```python
from build123d import *

# Parameters (mm, degrees)
F0_W     = 113.5
F0_H     = 50.5
F1_DEPTH = 215
F3_DEPTH = 113.501
F4_W     = 109.5
F4_H     = 18
F5_DEPTH = 43
F6_R     = 1.595
F7_DEPTH = 113.501
F8_R     = 1.595
F9_DEPTH = 10


with BuildPart() as f1:
    # F0 (on Top) → F1 (new body)
    with BuildSketch(Plane.XY):
        with Locations((56.75, 25.25)):
            Rectangle(F0_W, F0_H)
    extrude(amount=F1_DEPTH)

    # F2 (on face) → F3 (cut, through all)
    with BuildSketch(Plane.YZ.offset(113.5)):
        with BuildLine():
            Line((36.05, 209.85), (14.45, 209.85))
            ThreePointArc((14.45, 209.85), (13.38934, 209.41066), (12.95, 208.35))
            ThreePointArc((12.95, 208.35), (13.38934, 207.28934), (14.45, 206.85))
            Line((14.45, 206.85), (36.05, 206.85))
            ThreePointArc((36.05, 206.85), (37.11066, 207.28934), (37.55, 208.35))
            ThreePointArc((37.55, 208.35), (37.11066, 209.41066), (36.05, 209.85))
        make_face()
        with BuildLine():
            ThreePointArc((12.95, 201.35), (13.38934, 200.28934), (14.45, 199.85))
            Line((14.45, 199.85), (36.05, 199.85))
            ThreePointArc((36.05, 199.85), (37.11066, 200.28934), (37.55, 201.35))
            ThreePointArc((37.55, 201.35), (37.11066, 202.41066), (36.05, 202.85))
            Line((36.05, 202.85), (14.45, 202.85))
            ThreePointArc((14.45, 202.85), (13.38934, 202.41066), (12.95, 201.35))
        make_face()
        with BuildLine():
            ThreePointArc((12.95, 194.35), (13.38934, 193.28934), (14.45, 192.85))
            Line((14.45, 192.85), (36.05, 192.85))
            ThreePointArc((36.05, 192.85), (37.11066, 193.28934), (37.55, 194.35))
            ThreePointArc((37.55, 194.35), (37.11066, 195.41066), (36.05, 195.85))
            Line((36.05, 195.85), (14.45, 195.85))
            ThreePointArc((14.45, 195.85), (13.38934, 195.41066), (12.95, 194.35))
        make_face()
    extrude(amount=-F3_DEPTH, mode=Mode.SUBTRACT)

    # F4 (on face) → F5 (cut)
    with BuildSketch(Plane.XZ):
        with Locations((56.75, 206)):
            Rectangle(F4_W, F4_H)
    extrude(amount=-F5_DEPTH, mode=Mode.SUBTRACT)

    # F6 (on face) → F7 (cut, through all)
    with BuildSketch(Plane.YZ.offset(113.5)):
        with Locations((39.155, 31.595)):
            Circle(F6_R)
        with Locations((39.155, 182.905)):
            Circle(F6_R)
    extrude(amount=-F7_DEPTH, mode=Mode.SUBTRACT)

    # F8 (on face) → F9 (cut)
    with BuildSketch(Plane(origin=(0, 0, 0), x_dir=(0, -1, 0), z_dir=(-1, 0, 0))):
        with Locations((-13.345, 182.905)):
            Circle(F8_R)
        with Locations((-13.345, 31.595)):
            Circle(F8_R)
    extrude(amount=-F9_DEPTH, mode=Mode.SUBTRACT)


solid = f1.part
```
Can you work these out from the model? Positions are in its coordinate system, mm. A direction names the side the tool comes from. Give positions to 0.01 mm unless a question says otherwise; leave off trailing zeros. Order: outer loops, then holes, each group sorted by start corner. A loop starts at its lowest first (then second) coordinate and runs counter-clockwise, first axis right, second up. Notation, with made-up numbers: (-33, -29) - (-21, -29) arc R19 cw to (-21, -21) - close; hole circle Ø1 at (42.5, -22). An arc over 180 degrees is marked (long way). Use a Markdown table: item, result. Add a question column.
Q1. If we mould it in two halves opening along X, with no side actions, what happens to faces 1 (the flat face through (56, 21, 197)), 2 (the flat face through (58, 25, 195.85)), 3 (the flat face through (113.5, 25, 106))? For each: released by +X, released by -X, zero draft, split by the parting line, or undercut.
Q2. I'm going to push flat-ended pins straight in: pin 1 (1.6 mm diameter, centred on y = 13, z = 183, fed in from -X); pin 2 (6.5 mm diameter, centred on x = 44, y = 21.5, fed in from +Z). Where does each tip first touch, or does it pass through?
Q3. On a 3-axis mill with a long thin cutter (end or side, diameter ignored), from which of +Z, -Z, +X, -X, +Y, -Y can I reach the whole of each face in a straight line? I mean faces 4 (the flat face through (2, 21, 206)), 5 (the flat face through (0, 25, 106)), 6 (the flat face through (58, 25, 192.85)). Say none if no direction works.
Q4. If we section it at C-C on y = 4.5: Write out the boundary of the cut face in (x, z), plus the area to 3 significant figures.
Q5. Please list where these lines run through material, in increasing order: line 1 along X through (y, z) = (37.5, 202.5); line 2 along Z through (x, y) = (82.5, 35.5); line 3 along Z through (x, y) = (86, 38) (3 decimals).
Q6. If we section it at B-B on x = 53.5: Write out the boundary of the cut face in (y, z) (3 decimals), plus the area to 4 significant figures.
Q7. If we section it at A-A on y = 19.5: Write out the boundary of the cut face in (x, z).
Answers follow:
| question | item | result |
|---|---|---|
| 1 | face 1 | undercut |
| 1 | face 2 | zero draft |
| 1 | face 3 | released by +X |
| 2 | pin 1 | stops at x = 10 |
| 2 | pin 2 | stops at z = 197 |
| 3 | face 4 | +Z, -Y |
| 3 | face 5 | +Z, -Z, -X, +Y, -Y |
| 3 | face 6 | +X, -X |
| 4 | outline | (0, 0) - (113.5, 0) - (113.5, 215) - (111.5, 215) - (111.5, 197) - (2, 197) - (2, 215) - (0, 215) - close |
| 4 | area | 22,400 mm^2 |
| 5 | line 1 | x = 0 to 2, 111.5 to 113.5 |
| 5 | line 2 | z = 0 to 192.85, 195.85 to 197 |
| 5 | line 3 | z = 0 to 30.495, 32.695 to 181.805, 184.005 to 197 |
| 6 | outline | (0, 0) - (50.5, 0) - (50.5, 215) - (43, 215) - (43, 197) - (0, 197) - close; hole (12.95, 194.35) arc R1.5 ccw to (14.45, 192.85) - (36.05, 192.85) arc R1.5 ccw to (37.55, 194.35) arc R1.5 ccw to (36.05, 195.85) - (14.45, 195.85) arc R1.5 ccw to start; hole circle Ø3.19 at (39.155, 31.595); hole circle Ø3.19 at (39.155, 182.905) |
| 6 | area | 10,000 mm^2 |
| 7 | outline | (0, 0) - (113.5, 0) - (113.5, 192.85) - (0, 192.85) - close; (0, 195.85) - (113.5, 195.85) - (113.5, 199.85) - (111.5, 199.85) - (111.5, 197) - (2, 197) - (2, 199.85) - (0, 199.85) - close; (0, 202.85) - (2, 202.85) - (2, 206.85) - (0, 206.85) - close; (0, 209.85) - (2, 209.85) - (2, 215) - (0, 215) - close; (111.5, 202.85) - (113.5, 202.85) - (113.5, 206.85) - (111.5, 206.85) - close; (111.5, 209.85) - (113.5, 209.85) - (113.5, 215) - (111.5, 215) - close |
